```python
from build123d import *

# Parameters (mm, degrees)
F1_DEPTH    = 15.24
F3_DEPTH    = 3
F5_DEPTH    = 2.54
F6_DEPTH    = 6
F7_C1_SIZE2 = 3.81
F7_C1_SIZE  = 25.1924509954
F7_C2_SIZE2 = 3.81
F7_C2_SIZE  = 25.1924509954
F8_T1_DEPTH = 22.1165158115
F9_R        = 7.61999


# Not quite as in the source:
# - a fillet or chamfer that OpenCascade refuses, or shapes differently, is made with other operations: its cross-section is extruded or revolved along the edge and cut away or added
# - a fillet or chamfer is up to 0.001 mm smaller than in the source, because OpenCascade refuses the exact size


with BuildPart() as f1:
    # F0 (on Front) → F1 (new body)
    with BuildSketch(Plane.XZ):
        with BuildLine():
            ThreePointArc((-3, 4.5), (-3.4393398282, 3.4393398282), (-4.5, 3))
            Line((-4.5, 3), (-25.4, 3))
            Line((-25.4, 3), (-25.4, -3))
            Line((-25.4, -3), (-1.5, -3))
            ThreePointArc((-1.5, -3), (-0.4393398282, -2.5606601718), (0, -1.5))
            Line((0, -1.5), (0, 28.4))
            Line((0, 28.4), (-3, 28.4))
            Line((-3, 28.4), (-3, 4.5))
        make_face()
    extrude(amount=F1_DEPTH)

    # F2 (on face) → F3 (cut, through all)
    with BuildSketch(Plane.YZ):
        with BuildLine():
            ThreePointArc((-5.12, 23.4), (-7.62, 25.9), (-10.12, 23.4))
            Line((-10.12, 23.4), (-10.12, 9.5))
            ThreePointArc((-10.12, 9.5), (-7.62, 7), (-5.12, 9.5))
            Line((-5.12, 9.5), (-5.12, 23.4))
        make_face()
    extrude(amount=-F3_DEPTH, mode=Mode.SUBTRACT)

    # F4 (on face) → F5 (cut)
    with BuildSketch(Plane.XY.offset(3)):
        with BuildLine():
            ThreePointArc((-19.4, -3.57), (-23.45, -7.62), (-19.4, -11.67))
            Line((-19.4, -11.67), (-10.5, -11.67))
            ThreePointArc((-10.5, -11.67), (-6.45, -7.62), (-10.5, -3.57))
            Line((-10.5, -3.57), (-19.4, -3.57))
        make_face()
        with BuildLine():
            Line((-10.5, -10.12), (-19.4, -10.12))
            ThreePointArc((-19.4, -10.12), (-21.9, -7.62), (-19.4, -5.12))
            Line((-19.4, -5.12), (-10.5, -5.12))
            ThreePointArc((-10.5, -5.12), (-8, -7.62), (-10.5, -10.12))
        make_face(mode=Mode.SUBTRACT)
    extrude(amount=-F5_DEPTH, mode=Mode.SUBTRACT)

    # F6 (cut, through all): a face of the model
    f6_faces = [f1.faces().sort_by_distance(p)[0] for p in [
        (-14.95, -7.62, 3),
    ]]
    extrude(f6_faces, amount=-F6_DEPTH, mode=Mode.SUBTRACT)

    # F7: chamfer of 3.81 x 25.1924509954 on 2 edges, made by hand

    # F7_c1
    f7_c1_edges = [f1.edges().sort_by_distance(p)[0] for p in [
        (-1.5, 0, 28.4),
    ]]
    f7_c1_side = f1.faces().sort_by_distance((-1.5, 0, 28.3238))[0]
    chamfer(f7_c1_edges, length=F7_C1_SIZE, length2=F7_C1_SIZE2, reference=f7_c1_side)

    # F7_c2
    f7_c2_edges = [f1.edges().sort_by_distance(p)[0] for p in [
        (-1.5, -15.24, 28.4),
    ]]
    f7_c2_side = f1.faces().sort_by_distance((-1.5, -15.24, 28.3238))[0]
    chamfer(f7_c2_edges, length=F7_C2_SIZE, length2=F7_C2_SIZE2, reference=f7_c2_side)

    # F8: fillet of radius 4.445 on 2 edges, made by hand

    # F8_s2 → F8_t1 (cut)
    with BuildSketch(Plane.YZ.offset(-12.5582579057)):
        with BuildLine():
            ThreePointArc((-12.0017189515, 24.6196846016), (-10.5052742427, 27.3249071244), (-7.6066968377, 28.4))
            Line((-7.6066968377, 28.4), (-11.43, 28.4))
            Line((-11.43, 28.4), (-12.0017189515, 24.6196846016))
        make_face()
        with BuildLine():
            ThreePointArc((-3.2382810485, 24.6196846016), (-4.7347257573, 27.3249071244), (-7.6333031623, 28.4))
            Line((-7.6333031623, 28.4), (-3.81, 28.4))
            Line((-3.81, 28.4), (-3.2382810485, 24.6196846016))
        make_face()
    extrude(amount=F8_T1_DEPTH, mode=Mode.SUBTRACT)

    # F9 (radius 7.62 in the source; OpenCascade refuses exactly that, so slightly less here)
    f9_edges = [f1.edges().sort_by_distance(p)[0] for p in [
        (-25.4, -15.24, 0),
        (-25.4, 0, 0),
    ]]
    fillet(f9_edges, radius=F9_R)


solid = f1.part
```
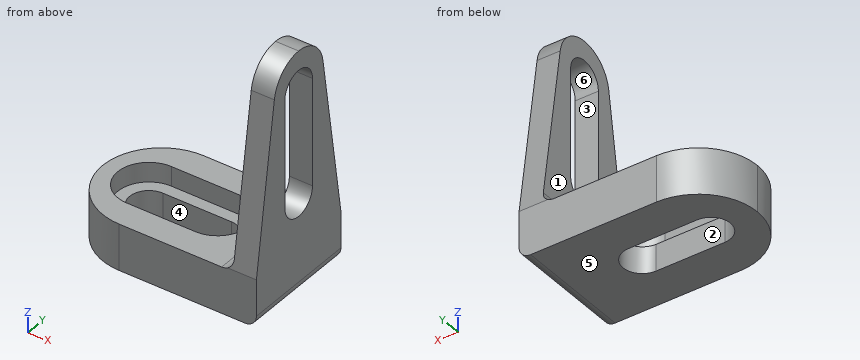
CAD build for the part. Positions are in the model's coordinates, mm. Face numbers are marked on the shaded views. A direction names the side the tool comes from. Coordinates: 2 decimals unless noted, no trailing zeros. Order: outer loops, then holes, each group sorted by start corner. A loop starts at its lowest first (then second) coordinate and runs counter-clockwise, first axis right, second up.
(1) Saw through at A-A, the plane x = -13. Write the cut outline in (y, z), and give its area (3 significant figures).
Solution:
outline: (-15.24, -3) - (-10.12, -3) - (-10.12, 0.46) - (-11.67, 0.46) - (-11.67, 3) - (-15.24, 3) - close; (-5.12, -3) - (0, -3) - (0, 3) - (-3.57, 3) - (-3.57, 0.46) - (-5.12, 0.46) - close
area: 53.6 mm2
(2) Mould opens along Z. For the marked faces 4, 5 and 6 say: released by +Z, released by -Z, zero draft, split by the parting line, or undercut.
Solution:
face 4: zero draft
face 5: released by -Z
face 6: undercut
(3) Saw through at D-D, the plane y = -1.25. Write the cut outline in (x, z).
Solution:
outline: (-21.96, -3) - (-1.5, -3) arc R1.5 ccw to (0, -1.5) - (0, 11.47) - (-3, 11.47) - (-3, 4.5) arc R1.5 cw to (-4.5, 3) - (-21.96, 3) - close
(4) Drill centre lines: L1, parallel to Y at x = -15.5, z = 2; L2, parallel to Y at x = -14.25, z = -1; L3, parallel to X at y = -13, z = 16. Where is each one in solid material? Low to high.
Solution:
L1: y = -15.24 to -11.67, -3.57 to 0
L2: y = -15.24 to -10.12, -5.12 to 0
L3: x = -3 to 0
(5) Saw through at C-C, the plane z = 21.5. Write the cut outline in (x, y).
Solution:
outline: (-3, -12.47) - (0, -12.47) - (0, -10.12) - (-3, -10.12) - close; (-3, -5.12) - (0, -5.12) - (0, -2.77) - (-3, -2.77) - close
(6) Which spindle directions (+Z, -Z, +X, -X, +Y, -Y) get a long thin tool onto all of the face, cutting with end or side? Do the marked faces 1, 2 and 3. Say none if no direction does.
Solution:
face 1: +Z, -X, +Y, -Y
face 2: +Z, -Z
face 3: +X, -X
(7) Saw through at B-B, the plane y = -6.5. Write the cut outline in (x, z), and give its area (3 significant figures).
Solution:
outline: (-25.32, -3) - (-21.64, -3) - (-21.64, 0.46) - (-23.29, 0.46) - (-23.29, 3) - (-25.32, 3) - close; (-8.26, -3) - (-1.5, -3) arc R1.5 ccw to (0, -1.5) - (0, 7.26) - (-3, 7.26) - (-3, 4.5) arc R1.5 cw to (-4.5, 3) - (-6.61, 3) - (-6.61, 0.46) - (-8.26, 0.46) - close; (-3, 25.64) - (0, 25.64) - (0, 28.25) - (-3, 28.25) - close
area: 83.9 mm2
(8) Pin check, flat tips, straight feed: pin 1 Ø5 at (x, z) = (-6.5, 10) entering from -Y; pin 2 Ø1.5 at (x, y) = (-16, -4.5) entering from +Z; pin 3 Ø4.5 at (y, z) = (-4.5, 20) entering from -X; pin 4 Ø0.9 at (x, z) = (-1.5, 13.5) entering from -Y. Stop position of each tip, or through.
Solution:
pin 1: passes through
pin 2: stops at z = 0.46
pin 3: stops at x = -3
pin 4: stops at y = -13.75
